The figure shows three views and two pictorial views of one solid part (mm, origin at its lowest corner). Answer the questions. Give positions to 0.01 mm unless a question says otherwise; leave off trailing zeros. Loops run counter-clockwise (first coordinate to the right, second up) from the corner with the lowest first, then second, coordinate; pieces in that order, holes last. Notation, with made-up numbers: (49, 44.25) - (79, 44.25) arc R11 cw to (79, 51.25) - close; hole circle Ø4 at (65.25, 34). An arc over 180 degrees is marked (long way). Write each question's results on one line, items separated by ' | '.
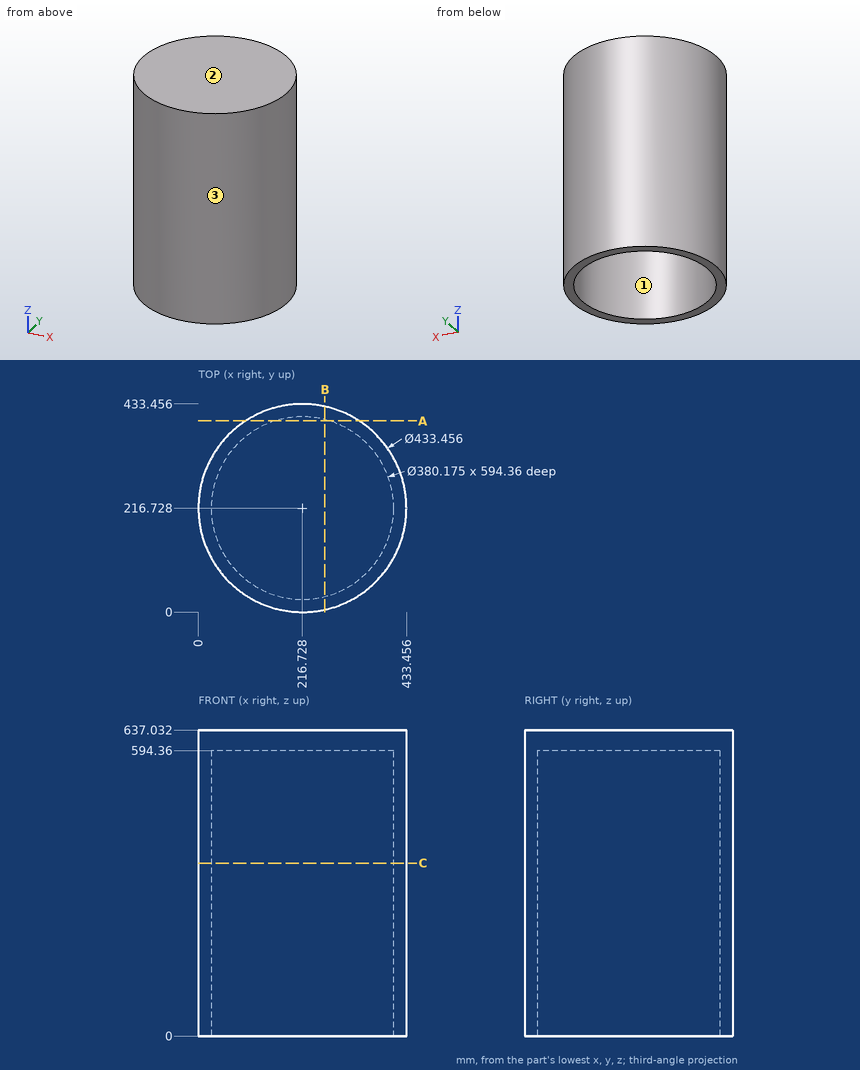
Item 1: A cutting plane is placed at B-B, the plane x = 263.5. Determine the outline of the cut face in (y, z) (1 decimal), plus the area to 3 significant figures.
Values found:
outline: (5.1, 0) - (32.5, 0) - (32.5, 594.4) - (401, 594.4) - (401, 0) - (428.3, 0) - (428.3, 637) - (5.1, 637) - close | area: 50,600 mm²
Item 2: A cutting plane is placed at A-A, the plane y = 398.5. Determine the outline of the cut face in (x, z) (1 decimal), plus the area to 3 significant figures.
Values found:
outline: (98.7, 0) - (161.1, 0) - (161.1, 594.4) - (272.3, 594.4) - (272.3, 0) - (334.8, 0) - (334.8, 637) - (98.7, 637) - close | area: 84,300 mm²
Item 3: Flat-ended cylindrical pins translate along their axes: P1, Ø12, axis at x = 307.5, z = 210, coming from the +Y side; P2, Ø1.5, axis at y = 297, z = 331.5, coming from the -X side; P3, Ø1.5, axis at y = 303.5, z = 527, coming from the +X side. Find the tip coordinate at first contact, or state that the pin passes through.
Values found:
P1: stops at y = 416.19 | P2: stops at x = 15.12 | P3: stops at x = 415.65
Item 4: Find the intervals of material crossed by line 1 along Y through (x, z) = (91, 496) (1 decimal); line 2 along Y through (x, z) = (211, 373) (1 decimal); line 3 along Z through (x, y) = (163, 55), in increasing order. Write a range as [from, to].
Values found:
line 1: y = [40.2, 74.2], [359.3, 393.3] | line 2: y = [0.1, 26.7], [406.7, 433.4] | line 3: z = [594.36, 637.03]
Item 5: For a pull along Y with two mould halves and no side action, classify the marked faces 1, 2 and 3 as released by +Y, released by -Y, zero draft, split by the parting line, or undercut.
Values found:
face 1: undercut | face 2: zero draft | face 3: split by the parting line
Item 6: A cutting plane is placed at C-C, the plane z = 360. Determine the outline of the cut face in (x, y) (1 decimal), plus the area to 3 significant figures.
Values found:
outline: circle Ø433.5 at (216.7, 216.7); hole circle Ø380.2 at (216.7, 216.7) | area: 34,000 mm²
